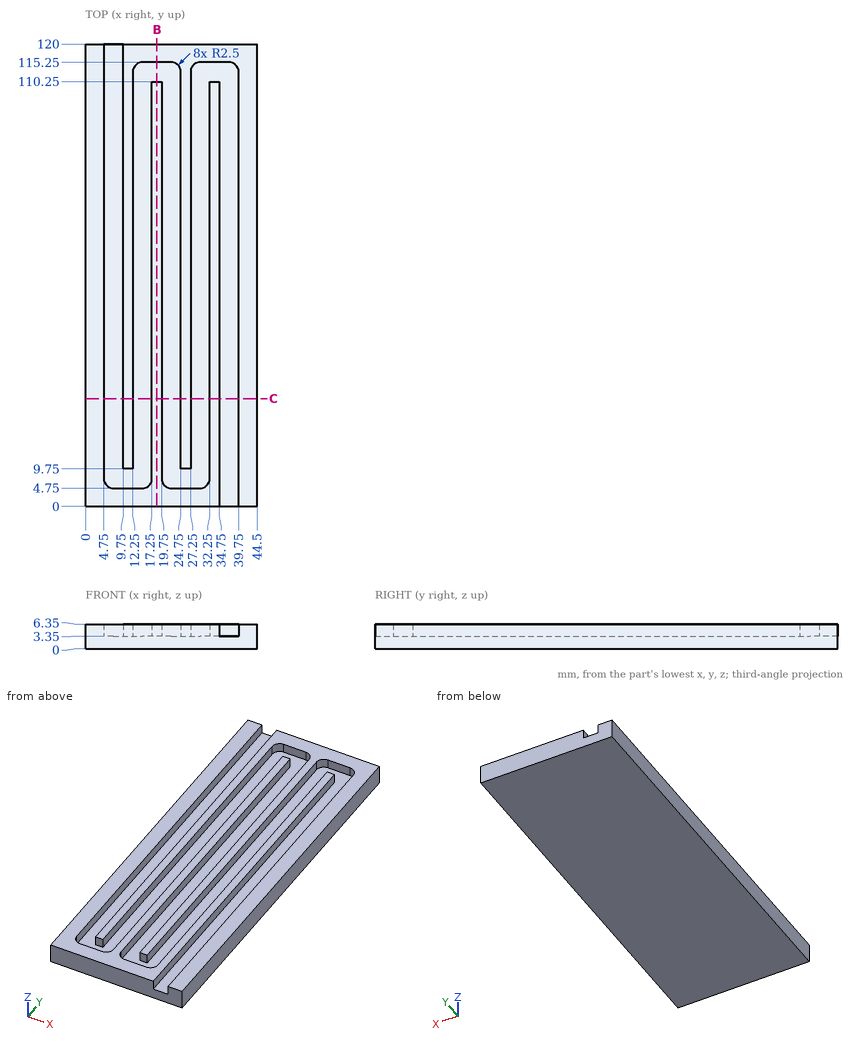
Could you check a few things on this drawing? It's one solid part, dimensions in mm from its lowest x, y, z. Coordinates: 2 decimals unless noted, no trailing zeros. Loops run counter-clockwise (first coordinate to the right, second up) from the corner with the lowest first, then second, coordinate; pieces in that order, holes last. Notation, with made-up numbers: (-29, 1.5) - (-9, 1.5) arc R18 cw to (-9, 32.5) - close; hole circle Ø1 at (-20.5, -5). An arc over 180 degrees is marked (long way). Return JSON: item names as keys, results as strings. Group by question number.
Item 1: I need wall thicknesses on line 1 (X direction, y = 10.5, z = 5.75); line 2 (Y direction, x = 17.5, z = 4); line 3 (Z direction, x = 5, y = 90.5). Which ranges of each line are inside material? Lowest first, please. Write a range as from..to.
Item 2: If we section it at B-B on x = 18.5: Write out the boundary of the cut face in (y, z), and give its area (3 significant figures).
Item 3: If we section it at C-C on y = 28: Write out the boundary of the cut face in (x, z), and give its area (3 significant figures).
Calculated:
{
 "1": {"line 1": "x = 0..4.75, 9.75..12.25, 17.25..19.75, 24.75..27.25, 32.25..34.75, 39.75..44.5", "line 2": "y = 0..110.25, 115.25..120", "line 3": "z = 0..3.35"},
 "2": {"outline": "(0, 0) - (120, 0) - (120, 6.35) - (115.25, 6.35) - (115.25, 3.35) - (110.25, 3.35) - (110.25, 6.35) - (0, 6.35) - close", "area": "747 mm^2"},
 "3": {"outline": "(0, 0) - (44.5, 0) - (44.5, 6.35) - (39.75, 6.35) - (39.75, 3.35) - (34.75, 3.35) - (34.75, 6.35) - (32.25, 6.35) - (32.25, 3.35) - (27.25, 3.35) - (27.25, 6.35) - (24.75, 6.35) - (24.75, 3.35) - (19.75, 3.35) - (19.75, 6.35) - (17.25, 6.35) - (17.25, 3.35) - (12.25, 3.35) - (12.25, 6.35) - (9.75, 6.35) - (9.75, 3.35) - (4.75, 3.35) - (4.75, 6.35) - (0, 6.35) - close", "area": "208 mm^2"}
}
